Check sheet for the modelled part. Datum: model origin and axes. Units: mm. Round coordinates to 2 decimals unless told otherwise and drop trailing zeros. Write each loop counter-clockwise with the first axis right and the second up, starting at its lowest first coordinate (ties: lowest second). Pieces come first, ordered by that corner, then holes.
Item 1: Cross-section at D-D on x = -109. Enter the section's corners in (y, z).
Item 2: Cross-section at C-C on z = 44. Enter the section's corners in (x, y), plus the area to 3 significant figures.
Item 3: Cross-section at B-B on y = -95. Enter the section's corners in (x, z), plus the area to 3 significant figures.
Item 4: Material ranges on line 1 (Z direction, x = -3.5, y = -201.5); line 2 (Y direction, x = 78.5, z = 34.5); line 3 (Y direction, x = 47.5, z = 23), recorded low to high.
Item 5: Go/stop test with flat-tipped pins: pin 1 Ø3 at (x, z) = (94.5, 37) entering from -Y; pin 2 Ø10 at (y, z) = (6.5, 15) entering from +X; pin 3 Ø2 at (y, z) = (132.5, 16) entering from +X. Record where each tip stops, or that it passes through.
from build123d import *

# Parameters (mm, degrees)
F0_W        = 250
F0_H        = 450
F1_DEPTH    = 50
F2_R        = 24.99999
F3_T1_DEPTH = 550.00001
F3_T3_DEPTH = 375


# Not quite as in the source:
# - a fillet or chamfer that OpenCascade refuses, or shapes differently, is made with other operations: its cross-section is extruded or revolved along the edge and cut away or added
# - a fillet or chamfer is up to 0.001 mm smaller than in the source, because OpenCascade refuses the exact size


with BuildPart() as f1:
    # F0 (on Top) → F1 (new body)
    with BuildSketch(Plane.XY):
        Rectangle(F0_W, F0_H)
    extrude(amount=F1_DEPTH)

    # F2 (radius 25 in the source; OpenCascade refuses exactly that, so slightly less here)
    f2_edges = [f1.edges().sort_by_distance(p)[0] for p in [
        (-125, -225, 25),
        (125, -225, 25),
        (0, -225, 0),
        (0, -225, 50),
    ]]
    fillet(f2_edges, radius=F2_R)

    # F3: fillet of radius 25 on 4 edges, made by hand

    # F3_s2 → F3_t1 (cut)
    with BuildSketch(Plane.XZ.offset(-287.5)):
        with BuildLine():
            ThreePointArc((-125, 25), (-117.6776695297, 7.3223304703), (-100, 0))
            Line((-100, 0), (-125, 0))
            Line((-125, 0), (-125, 25))
        make_face()
        with BuildLine():
            ThreePointArc((100, 0), (117.6776695297, 7.3223304703), (125, 25))
            Line((125, 25), (125, 0))
            Line((125, 0), (100, 0))
        make_face()
    extrude(amount=F3_T1_DEPTH, mode=Mode.SUBTRACT)

    # F3_s4 → F3_t3 (cut)
    with BuildSketch(Plane.YZ.offset(-187.5)):
        with BuildLine():
            ThreePointArc((200, 0), (217.6776695297, 7.3223304703), (225, 25))
            Line((225, 25), (225, 0))
            Line((225, 0), (200, 0))
        make_face()
    extrude(amount=F3_T3_DEPTH, mode=Mode.SUBTRACT)


solid = f1.part
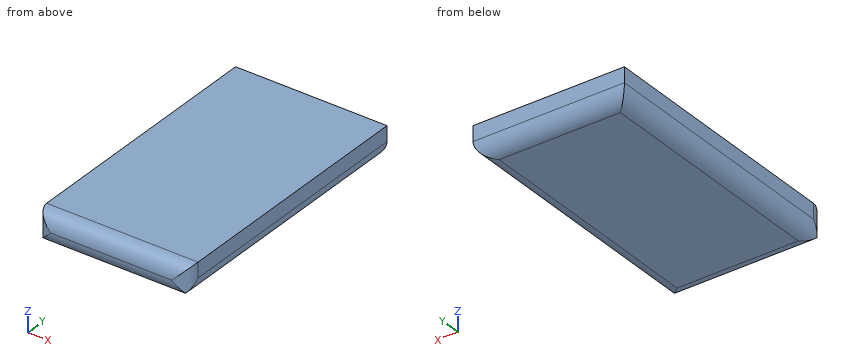
Response values:
1. outline: (-223.32, 16) arc R25 ccw to (-209, 1.68) - (209, 1.68) arc R25 ccw to (225, 25) - (225, 50) - (-200, 50) arc R25 ccw to (-223.32, 34) - close
2. outline: (-125, -200) arc R25 ccw to (-119, -216.25) - (119, -216.25) arc R25 ccw to (125, -200) - (125, 225) - (-125, 225) - close
2. area: 110,000 mm2
3. outline: (-125, 25) arc R25 ccw to (-100, 0) - (100, 0) arc R25 ccw to (125, 25) - (125, 50) - (-125, 50) - close
3. area: 12,200 mm2
4. line 1: z = 0.05 to 49.95
4. line 2: y = -223.12 to 225
4. line 3: y = -224.92 to 224.92
5. pin 1: stops at y = -222.69
5. pin 2: stops at x = 124.49
5. pin 3: stops at x = 123.69
